Could you check a few things on this model? Use its own coordinates, in mm. A direction names the side the tool comes from. Round coordinates to 2 decimals unless told otherwise and drop trailing zeros. Loops run counter-clockwise (first coordinate to the right, second up) from the corner with the lowest first, then second, coordinate; pieces in that order, holes last. Notation, with made-up numbers: M -5,-11.5 L 1,-11.5 A23 cw 1,9.5 Z; hole C 3.5,82 d10. An arc over 180 degrees is marked long. Return JSON: item names as keys, results as strings. Group by question number.
```python
from build123d import *

# Parameters (mm, degrees)
SKETCH1_R                      = 5
BOSS_EXTRUDE1_DEPTH            = 14
CHAMFER1_SIZE                  = 0.5
CUT_EXTRUDE1_REACH             = 16
SKETCH2_R                      = 0.75
SKETCH3_W                      = 5
SKETCH3_H                      = 10
CUT_EXTRUDE2_DEPTH             = 7
CUT_EXTRUDE3_REACH             = 7
SKETCH4_R                      = 0.75
CUT_EXTRUDE3_DIRECTION_2_REACH = 7


with BuildPart() as part:
    # Sketch1 → Boss-Extrude1 (new body)
    with BuildSketch(Plane(origin=(0, 0, 0), x_dir=(1, 0, 0), z_dir=(0, 1, 0))):
        Circle(SKETCH1_R)
    extrude(amount=BOSS_EXTRUDE1_DEPTH)

    # Chamfer1
    chamfer1_edges = [part.edges().sort_by_distance(p)[0] for p in [
        (-5, 0, 0),
        (-5, 14, 0),
    ]]
    chamfer(chamfer1_edges, length=CHAMFER1_SIZE)

    # Sketch2 → Cut-Extrude1 (cut, up to next)
    with BuildSketch(Plane.XZ, mode=Mode.PRIVATE) as cut_extrude1_sk1:
        Circle(SKETCH2_R)
    cut_extrude1_tool1 = extrude(cut_extrude1_sk1.sketch, amount=-CUT_EXTRUDE1_REACH, mode=Mode.PRIVATE) & part.part
    add(cut_extrude1_tool1.solids().sort_by_distance((0, 0, 0))[0], mode=Mode.SUBTRACT)

    # Sketch3 → Cut-Extrude2 (cut)
    with BuildSketch(Plane(origin=(0, 14, 0), x_dir=(1, 0, 0), z_dir=(0, 1, 0))):
        Rectangle(SKETCH3_W, SKETCH3_H)
    extrude(amount=-CUT_EXTRUDE2_DEPTH, mode=Mode.SUBTRACT)

    # Sketch4 → Cut-Extrude3 (cut, up to next)
    with BuildSketch(Plane(origin=(0, 0, 0), x_dir=(0, 0, -1), z_dir=(1, 0, 0)), mode=Mode.PRIVATE) as cut_extrude3_sk1:
        with Locations((0, 10.75)):
            Circle(SKETCH4_R)
    cut_extrude3_tool1 = extrude(cut_extrude3_sk1.sketch, amount=-CUT_EXTRUDE3_REACH, mode=Mode.PRIVATE) & part.part
    add(cut_extrude3_tool1.solids().sort_by_distance((0, 10.75, 0))[0], mode=Mode.SUBTRACT)

    # Sketch4 → Cut-Extrude3 direction 2 (cut, up to next)
    with BuildSketch(Plane(origin=(0, 0, 0), x_dir=(0, 0, -1), z_dir=(1, 0, 0)), mode=Mode.PRIVATE) as cut_extrude3_direction_2_sk1:
        with Locations((0, 10.75)):
            Circle(SKETCH4_R)
    cut_extrude3_direction_2_tool1 = extrude(cut_extrude3_direction_2_sk1.sketch, amount=CUT_EXTRUDE3_DIRECTION_2_REACH, mode=Mode.PRIVATE) & part.part
    add(cut_extrude3_direction_2_tool1.solids().sort_by_distance((0, 10.75, 0))[0], mode=Mode.SUBTRACT)


solid = part.part
```
1. If we section it at C-C, the plane y = 11.25: Please give me the cut outline in (x, z).
2. I need wall thicknesses on probe 1 along Z at (x, y) = (0, 1.5); probe 2 along Y at (x, z) = (-4.35, 0); probe 3 along Y at (x, z) = (-1, 0). Which ranges of each line are inside material? Lowest first, please.
3. We'd pull the mould along X, two halves only. Please class faces 1 (the face through (2.5, 9.8, 0.1)), 2 (the face through (-4.635, 13.865, -0.068)), 3 (the face through (4.635, 13.865, 0.068)), 4 (the face through (-0.75, 3.45, 0.03)): +X half, -X half, draft (parallel to the pull), parting line (faces both ways), or undercut.
4. I'm going to push flat-ended pins straight in: pin 1 Ø2 at (y, z) = (9, -2) entering from -X; pin 2 Ø2 at (y, z) = (2.5, 0.5) entering from -X; pin 3 Ø4 at (y, z) = (4.5, -4) entering from +X; pin 4 Ø1 at (y, z) = (1.5, -4) entering from -X. Where does each tip first touch, or does it pass through?
5. If we section it at D-D, the plane y = 2.75: Please give me the cut outline in (x, z), then the cut area to 3 significant figures.
6. If we section it at B-B, the plane z = 0: Please give me the cut outline in (x, y).
7. If we section it at A-A, the plane x = 0: Please give me the cut outline in (y, z).
8. On a 3-axis mill with a long thin cutter (end or side, diameter ignored), from which of +Z, -Z, +X, -X, +Y, -Y can I reach the whole of each face in a straight line? I mean faces 5 (the face through (3, 14, 0)), 6 (the face through (-2.5, 9.8, 0.1)). Say none if no direction works.
Geometry results:
{
 "1": {"outline": "M -4.97,-0.56 A5 ccw -2.5,-4.33 L -2.5,-0.56 Z; M -4.97,0.56 L -2.5,0.56 L -2.5,4.33 A5 ccw Z; M 2.5,-4.33 A5 ccw 4.97,-0.56 L 2.5,-0.56 Z; M 2.5,0.56 L 4.97,0.56 A5 ccw 2.5,4.33 Z"},
 "2": {"probe 1": "-5 to -0.75, 0.75 to 5", "probe 2": "0 to 10, 11.5 to 14", "probe 3": "0 to 7"},
 "3": {"face 1": "undercut", "face 2": "-X half", "face 3": "+X half", "face 4": "undercut"},
 "4": {"pin 1": "x = -4.9", "pin 2": "x = -5", "pin 3": "x = 4.58", "pin 4": "x = -3.57"},
 "5": {"outline": "C 0,0 d10; hole C 0,0 d1.5", "area": "76.8 mm^2"},
 "6": {"outline": "M -5,0.5 L -4.5,0 L -0.75,0 L -0.75,7 L -2.5,7 L -2.5,10 L -5,10 Z; M -5,11.5 L -2.5,11.5 L -2.5,14 L -4.5,14 L -5,13.5 Z; M 0.75,0 L 4.5,0 L 5,0.5 L 5,10 L 2.5,10 L 2.5,7 L 0.75,7 Z; M 2.5,11.5 L 5,11.5 L 5,13.5 L 4.5,14 L 2.5,14 Z"},
 "7": {"outline": "M 0,-4.5 L 0.5,-5 L 7,-5 L 7,-0.75 L 0,-0.75 Z; M 0,0.75 L 7,0.75 L 7,5 L 0.5,5 L 0,4.5 Z"},
 "8": {"face 5": "+Z, -Z, +X, -X, +Y", "face 6": "+Z, -Z, +Y"}
}
